Geometry check sheet. Reference: drawing and pictorial views, mm from the part's lowest x, y, z. Coordinates: 2 decimals unless noted, no trailing zeros. Loops run counter-clockwise (first coordinate to the right, second up) from the corner with the lowest first, then second, coordinate; pieces in that order, holes last. Notation, with made-up numbers: (45, 64) -> (76, 64) arc R26 cw to (76, 101) -> close; hole circle Ø8 at (10, 34.25). An arc over 180 degrees is marked (long way). Answer as a JSON object with one key per item and string values. Group by question number.
Q1. Cross-section at B-B on x = 77. Record the boundary of the cut face in (y, z), and give its area (3 significant figures).
Q2. Gauge pin test, flat end, axial feed: pin 1 Ø1.8 at (x, z) = (5, 52) entering from +Y. Record the tip position at first contact, or that the pin passes through.
Q3. Cross-section at A-A on z = 19. Record the boundary of the cut face in (x, y), and give its area (3 significant figures).
Q4. Scan lines: L1, parallel to Z at x = 98, y = 4; L2, parallel to X at y = 2, z = 10; L3, parallel to Z at x = 65, y = 3.4. Record each from-to range of solid material in increasing order.
Q5. Cross-section at D-D on y = 3.8. Record the boundary of the cut face in (x, z), and give its area (3 significant figures).
Q6. Cross-section at C-C on x = 98. Record the boundary of the cut face in (y, z).
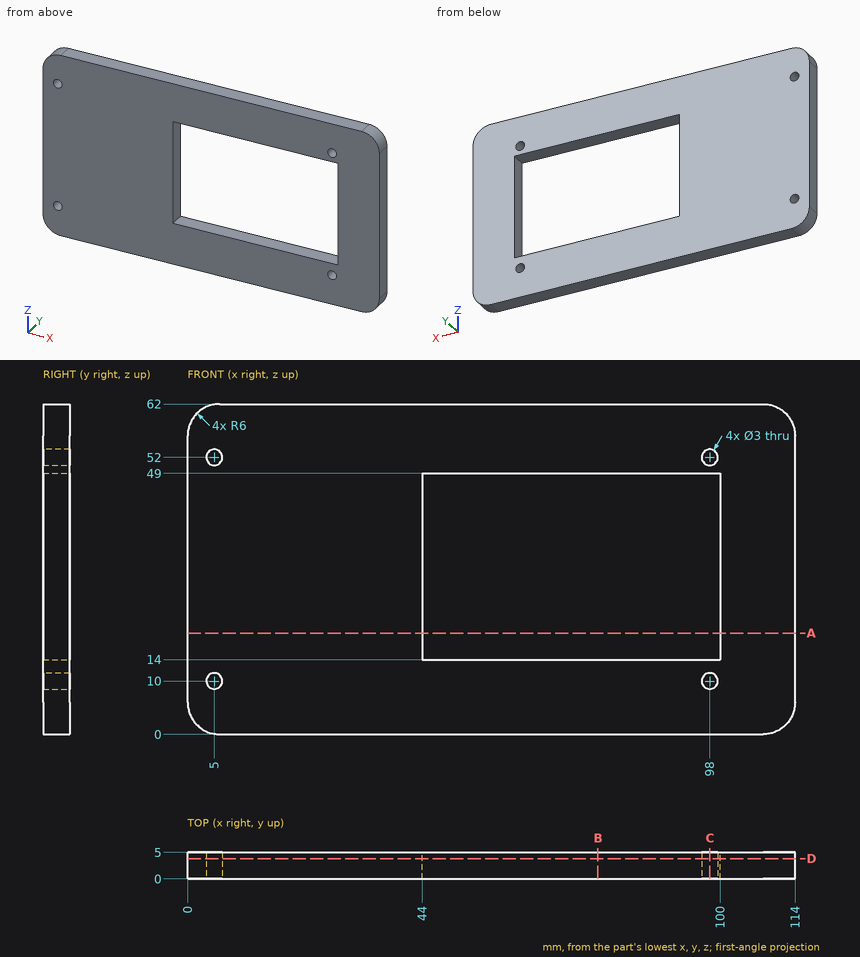
Computed values:
{
 "1": {"outline": "(0, 0) -> (5, 0) -> (5, 14) -> (0, 14) -> close; (0, 49) -> (5, 49) -> (5, 62) -> (0, 62) -> close", "area": "135 mm²"},
 "2": {"pin 1": "passes through"},
 "3": {"outline": "(0, 0) -> (44, 0) -> (44, 5) -> (0, 5) -> close; (100, 0) -> (114, 0) -> (114, 5) -> (100, 5) -> close", "area": "290 mm²"},
 "4": {"L1": "z = 0 to 8.5, 11.5 to 14, 49 to 50.5, 53.5 to 62", "L2": "x = 0 to 3.5, 6.5 to 96.5, 99.5 to 114", "L3": "z = 0 to 14, 49 to 62"},
 "5": {"outline": "(0, 6) arc R6 ccw to (6, 0) -> (108, 0) arc R6 ccw to (114, 6) -> (114, 56) arc R6 ccw to (108, 62) -> (6, 62) arc R6 ccw to (0, 56) -> close; hole circle Ø3 at (5, 10); hole circle Ø3 at (5, 52); hole (44, 14) -> (100, 14) -> (100, 49) -> (44, 49) -> close; hole circle Ø3 at (98, 10); hole circle Ø3 at (98, 52)", "area": "5,050 mm²"},
 "6": {"outline": "(0, 0) -> (5, 0) -> (5, 8.5) -> (0, 8.5) -> close; (0, 11.5) -> (5, 11.5) -> (5, 14) -> (0, 14) -> close; (0, 49) -> (5, 49) -> (5, 50.5) -> (0, 50.5) -> close; (0, 53.5) -> (5, 53.5) -> (5, 62) -> (0, 62) -> close"}
}
